Can you work these out from the drawing? Everything is in mm from the part's minimum corner. Coordinates: 2 decimals unless noted, no trailing zeros. Order: outer loops, then holes, each group sorted by start corner. A loop starts at its lowest first (then second) coordinate and runs counter-clockwise, first axis right, second up. Notation, with made-up numbers: M 11,36 L 31,36 A29 cw 31,73 Z; hole C 34.5,-10.75 d11. An arc over 180 degrees is marked long. Answer as a JSON object with one key per item and string values.
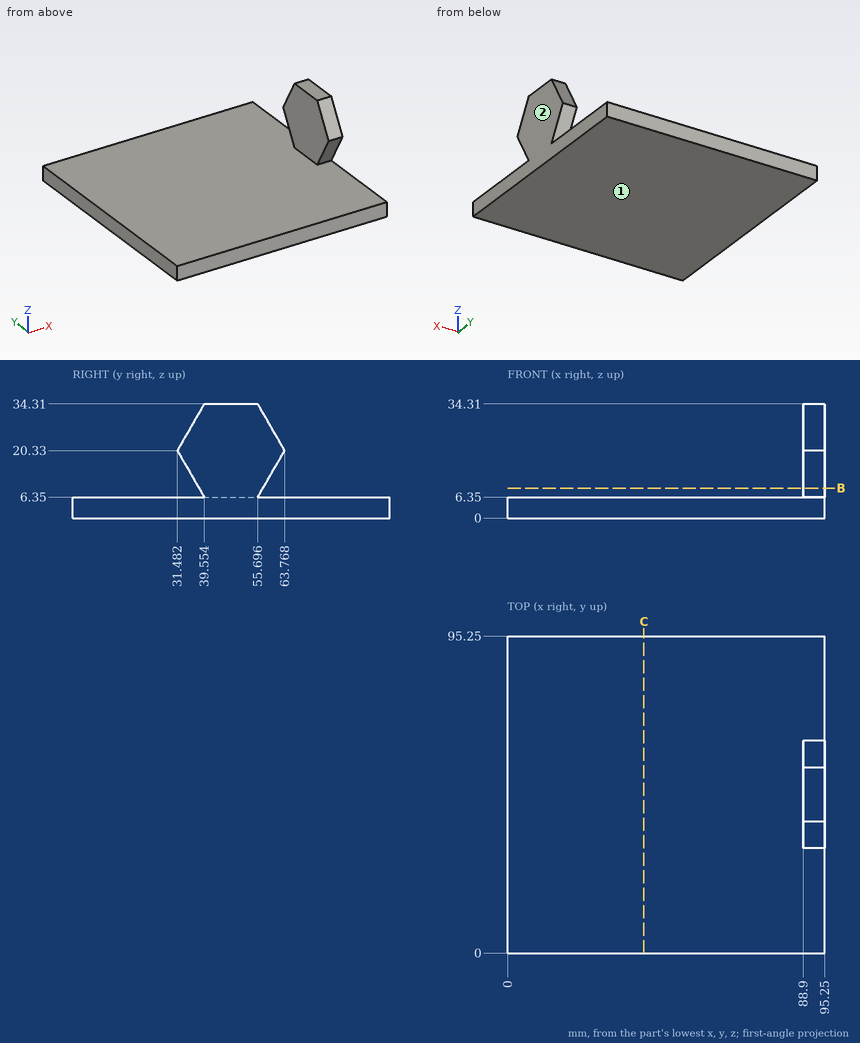
Item 1: I want a section at C-C, the plane x = 41. Write out the boundary of the cut face in (y, z).
Answers follow:
{"outline": "M 0,0 L 95.25,0 L 95.25,6.35 L 0,6.35 Z"}
Item 2: If we mould it in two halves opening along Z, with no side actions, what happens to the marked faces 1 and 2? For each: pulls with the +Z half, pulls with the -Z half, needs draft (parallel to the pull), parting line crosses it, or undercut.
Answers follow:
{"face 1": "pulls with the -Z half", "face 2": "needs draft"}
Item 3: I want a section at B-B, the plane z = 9. Write out the boundary of the cut face in (x, y).
Answers follow:
{"outline": "M 88.9,38.02 L 95.25,38.02 L 95.25,57.23 L 88.9,57.23 Z"}
Item 4: Please list where these lines run through material, in increasing order: line 1 (Z direction, x = 74, y = 50); line 2 (X direction, y = 41.5, z = 28); line 3 (Y direction, x = 89, z = 14.5).
Answers follow:
{"line 1": "z = 0 to 6.35", "line 2": "x = 88.9 to 95.25", "line 3": "y = 34.85 to 60.4"}
Item 5: I'm going to push flat-ended pins straight in: pin 1 (2 mm diameter, centred on x = 45, z = 6, fed in from -Y); pin 2 (8.5 mm diameter, centred on y = 55, z = 21, fed in from -X). Where does each tip first touch, or does it pass through?
Answers follow:
{"pin 1": "stops at y = 0", "pin 2": "stops at x = 88.9"}
